```python
from build123d import *

# Parameters (mm, degrees)
F1_DEPTH = 5
F2_R     = 5
F3_DEPTH = 10
F4_R     = 2.5
F4_R_2   = 1.5
F5_DEPTH = 45
F7_DEPTH = 25


with BuildPart() as f1:
    # F0 (on Top) → F1 (new body)
    with BuildSketch(Plane.XY):
        Polygon((-45, 0), (0, 0), (0, 5), (-35, 5), (-40, 10), (-10, 10), (-15, 15), (-40, 15), (-40, 20), (0, 20), (0, 25), (-45, 25), align=None)
    extrude(amount=F1_DEPTH)

    # F2 (on face) → F3 (join)
    with BuildSketch(Plane(origin=(-45, 0, 0), x_dir=(0, -1, 0), z_dir=(-1, 0, 0))):
        with Locations((-13, 2.5)):
            Circle(F2_R)
    extrude(amount=F3_DEPTH)

    # F4 (on face) → F5 (join)
    with BuildSketch(Plane(origin=(-55, 0, 0), x_dir=(0, -1, 0), z_dir=(-1, 0, 0))):
        with Locations((-13, 2.5)):
            Circle(F4_R)
        with Locations((-13, 2.5)):
            Circle(F4_R_2, mode=Mode.SUBTRACT)
    extrude(amount=F5_DEPTH)

    # F6 (on face) → F7 (cut)
    with BuildSketch(Plane.XZ):
        Polygon((-100.207202, 5.022824), (-100.207202, 0), (-88.150322, 5.022824), align=None)
    extrude(amount=-F7_DEPTH, mode=Mode.SUBTRACT)


solid = f1.part
```
The listing builds one solid part. Answer for the finished solid, in the listing's coordinates (mm). A direction names the side the tool comes from. Round coordinates to 2 decimals unless told otherwise and drop trailing zeros. Loops run counter-clockwise (first coordinate to the right, second up) from the corner with the lowest first, then second, coordinate; pieces in that order, holes last.
Q1. Section C-C, the plane z = 2.5 is taken. Determine the outline of the cut face in (x, y).
Q2. Find the intervals of material crossed by line 1 (Y direction, x = -69, z = 2.5); line 2 (Y direction, x = -16, z = 3.5); line 3 (Z direction, x = -87, y = 13), in increasing order.
Q3. Section A-A, the plane x = -30 is taken. Determine the outline of the cut face in (y, z).
Q4. Given pin 1 Ø2 at (x, y) = (-36, 21.5) entering from +Z; pin 2 Ø2.5 at (y, z) = (22.5, 2.5) entering from -X; pin 3 Ø1.5 at (y, z) = (17.5, 2) entering from +X, each flat-ended and moving along its own axis, determine where each tip first touches the part or whether it passes through.
Q5. Section B-B, the plane x = -7 is taken. Determine the outline of the cut face in (y, z).
Q6. For a pull along Y with two mould halves and no side action, classify faces 1 (the face through (-55, 13, 3)), 2 (the face through (-77.18, 13.54, 0.06)), 3 (the face through (-45, 21, 2)) as released by +Y, released by -Y, zero draft, split by the parting line, or undercut.
Q7. Which of the six approach directions +Z, -Z, +X, -X, +Y, -Y give full straight-line access (tool end or side, diameter ignored) to faces 4 (the face through (-45, 13, -1)), 5 (the face through (-49.93, 8.23, 4)), 6 (the face through (-45, 13, 6)), 7 (the face through (-17, 5, 2)), 8 (the face through (0, 2, 2))?
Q8. Section D-D, the plane y = 4 is taken. Determine the outline of the cut face in (x, z), then the cut area to 3 significant figures.
Completed:
1. outline: (-94.21, 10.5) - (-55, 10.5) - (-55, 8) - (-45, 8) - (-45, 0) - (0, 0) - (0, 5) - (-35, 5) - (-40, 10) - (-10, 10) - (-15, 15) - (-40, 15) - (-40, 20) - (0, 20) - (0, 25) - (-45, 25) - (-45, 18) - (-55, 18) - (-55, 15.5) - (-94.21, 15.5) - (-94.21, 14.5) - (-55, 14.5) - (-55, 11.5) - (-94.21, 11.5) - close
2. line 1: y = 10.5 to 11.5, 14.5 to 15.5
2. line 2: y = 0 to 5, 10 to 15, 20 to 25
2. line 3: z = 0 to 1, 4 to 5
3. outline: (0, 0) - (5, 0) - (5, 5) - (0, 5) - close; (10, 0) - (15, 0) - (15, 5) - (10, 5) - close; (20, 0) - (25, 0) - (25, 5) - (20, 5) - close
4. pin 1: stops at z = 5
4. pin 2: stops at x = -45
4. pin 3: stops at x = -40
5. outline: (0, 0) - (5, 0) - (5, 5) - (0, 5) - close; (20, 0) - (25, 0) - (25, 5) - (20, 5) - close
6. face 1: undercut
6. face 2: split by the parting line
6. face 3: zero draft
7. face 4: -Z, +X, +Y, -Y
7. face 5: -X
7. face 6: +Z, +X, +Y, -Y
7. face 7: +Z, -Z, +X
7. face 8: +Z, -Z, +X, +Y, -Y
8. outline: (-45, 0) - (0, 0) - (0, 5) - (-45, 5) - close
8. area: 225 mm2
